The drawing under review shows one solid part. Ordinate dimensions are in mm from its lowest x, y, z. Coordinates: 2 decimals unless noted, no trailing zeros. Write each loop counter-clockwise with the first axis right and the second up, starting at its lowest first coordinate (ties: lowest second). Pieces come first, ordered by that corner, then holes. Notation, with made-up numbers: M 64.25,65 L 84.25,65 A22 cw 84.25,95 Z; hole C 89.5,75.5 d1. An arc over 180 degrees is marked long. Write item = value, one per line.
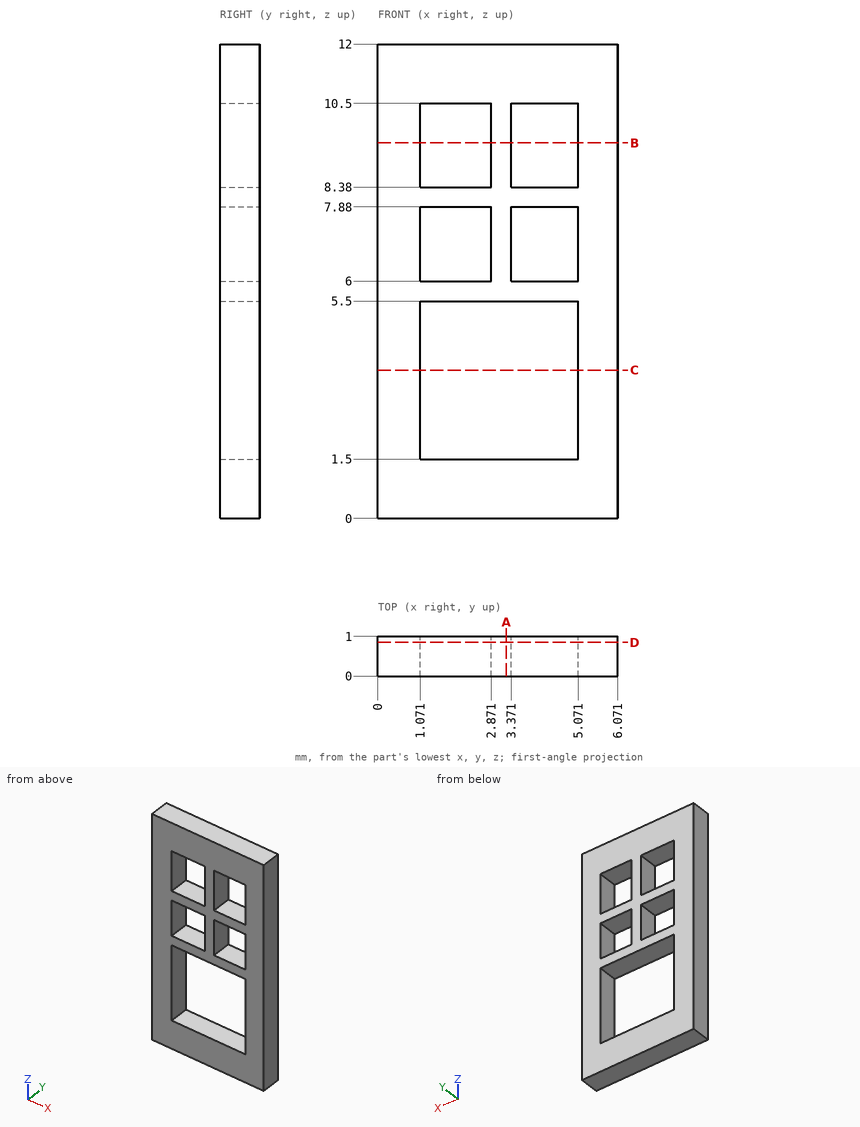
Q1. Consider section C-C, the plane z = 3.75. State the section outline as (x, y) points.
Check result:
outline = M 0,0 L 1.07,0 L 1.07,1 L 0,1 Z; M 5.07,0 L 6.07,0 L 6.07,1 L 5.07,1 Z
Q2. Consider section B-B, the plane z = 9.5. State the section outline as (x, y) points.
Check result:
outline = M 0,0 L 1.07,0 L 1.07,1 L 0,1 Z; M 2.87,0 L 3.37,0 L 3.37,1 L 2.87,1 Z; M 5.07,0 L 6.07,0 L 6.07,1 L 5.07,1 Z
Q3. Wall thickness on line 1 (Z direction, x = 2.25, y = 0.3); line 2 (X direction, y = 0.95, z = 10.25); line 3 (X direction, y = 0.85, z = 2): over which ranges is each line inside the solid? List them lowest first.
Check result:
line_1 = 0 to 1.5, 5.5 to 6, 7.88 to 8.38, 10.5 to 12
line_2 = 0 to 1.07, 2.87 to 3.37, 5.07 to 6.07
line_3 = 0 to 1.07, 5.07 to 6.07
Q4. Consider section D-D, the plane y = 0.85. State the section outline as (x, z) points.
Check result:
outline = M 0,0 L 6.07,0 L 6.07,12 L 0,12 Z; hole M 1.07,1.5 L 5.07,1.5 L 5.07,5.5 L 1.07,5.5 Z; hole M 1.07,6 L 2.87,6 L 2.87,7.88 L 1.07,7.88 Z; hole M 1.07,8.38 L 2.87,8.38 L 2.87,10.5 L 1.07,10.5 Z; hole M 3.37,6 L 5.07,6 L 5.07,7.88 L 3.37,7.88 Z; hole M 3.37,8.38 L 5.07,8.38 L 5.07,10.5 L 3.37,10.5 Z
Q5. Consider section A-A, the plane x = 3.25. State the section outline as (y, z) points.
Check result:
outline = M 0,0 L 1,0 L 1,1.5 L 0,1.5 Z; M 0,5.5 L 1,5.5 L 1,12 L 0,12 Z
